from build123d import *

# Parameters (mm, degrees)
SKETCH_1_R           = 3.5
EXTRUDE_1_DEPTH      = 3
SKETCH_2_R           = 1.5
CUT_EXTRUDE_1_DEPTH  = 10
EXTRUDE_2_DEPTH      = 4
EXTRUDE_5_DEPTH      = 7
FILLET_1_R           = 2
HOLE_WIZARD_M2_5_1_D = 2.05
SKETCH_12_R          = 4.953561737
SKETCH_12_R_2        = 3.03
EXTRUDE_6_DEPTH      = 3


with BuildPart() as part:
    # 草图1 → 凸台-拉伸1 (new body)
    with BuildSketch(Plane.XY):
        with BuildLine():
            Line((0, 0), (17, 0))
            Line((17, 0), (17, 21))
            ThreePointArc((17, 21), (14.559389791, 26.961023013), (8.639106973, 29.498861644))
            ThreePointArc((8.639106973, 29.498861644), (4.214678609, 30.921411086), (1.327625741, 34.563407653))
            ThreePointArc((1.327625741, 34.563407653), (-5.234705957, 62.223549547), (-3.748501306, 90.612611571))
            ThreePointArc((-3.748501306, 90.612611571), (-5.162788524, 92.923505905), (-7.58241645, 91.704554856))
            ThreePointArc((-7.58241645, 91.704554856), (-12.196269834, 55.45091149), (0, 21))
            Line((0, 21), (0, 0))
        make_face()
        with Locations((8.5, 21)):
            Circle(SKETCH_1_R, mode=Mode.SUBTRACT)
    extrude(amount=EXTRUDE_1_DEPTH)

    # 草图2 → 切除-拉伸1 (cut)
    with BuildSketch(Plane(origin=(0, 0, 0), x_dir=(-1, 0, 0), z_dir=(0, 0, -1))):
        with Locations((-14, 4)):
            Circle(SKETCH_2_R)
        with Locations(Location((-3, 4, 0), (0, 0, 180))):
            Circle(SKETCH_2_R)
    extrude(amount=-CUT_EXTRUDE_1_DEPTH, mode=Mode.SUBTRACT)

    # 草图3 → 凸台-拉伸2 (add)
    with BuildSketch(Plane.XY.offset(3)):
        with BuildLine():
            ThreePointArc((-7.58241645, 91.704554856), (-12.6426678, 63.080202535), (-7.007767698, 34.563407653))
            Line((-7.007767698, 34.563407653), (1.327625741, 34.563407653))
            ThreePointArc((1.327625741, 34.563407653), (-5.234705957, 62.223549547), (-3.748501306, 90.612611571))
            ThreePointArc((-3.748501306, 90.612611571), (-5.162788524, 92.923505905), (-7.58241645, 91.704554856))
        make_face()
    extrude(amount=EXTRUDE_2_DEPTH)

    # 草图8 → 凸台-拉伸5 (add)
    with BuildSketch(Plane(origin=(0, 0, 0), x_dir=(-1, 0, 0), z_dir=(0, 0, -1))):
        with BuildLine():
            Line((8.353336216, 89.563407653), (13.622203114, 89.563407653))
            ThreePointArc((13.622203114, 89.563407653), (17.624786926, 61.957713987), (12.366747323, 34.563407653))
            Line((12.366747323, 34.563407653), (7.007767698, 34.563407653))
            ThreePointArc((7.007767698, 34.563407653), (12.623031035, 61.942490485), (8.353336216, 89.563407653))
        make_face()
    extrude(amount=-EXTRUDE_5_DEPTH)

    # 圆角1
    fillet_1_edges = [part.edges().sort_by_distance(p)[0] for p in [
        (-12.366747323, 34.563407653, 3.5),
        (-13.622203114, 89.563407653, 3.5),
        (-8.353336216, 89.563407653, 3.5),
        (-7.007767698, 34.563407653, 1.5),
    ]]
    fillet(fillet_1_edges, radius=FILLET_1_R)

    # M2.5 螺纹孔1 (through all)
    with Locations(Plane(origin=(0, 0, 0), x_dir=(-1, 0, 0), z_dir=(0, 0, -1))):
        with Locations((14.33753876, 52.418963936), (-20.3596947, 65.689324708), (13.008857265, 82.418963936), (15.069556912, 67.418963936)):
            Hole(HOLE_WIZARD_M2_5_1_D / 2)

    # 草图12 → 凸台-拉伸6 (add)
    with BuildSketch(Plane(origin=(0, 0, 0), x_dir=(-1, 0, 0), z_dir=(0, 0, -1))):
        with Locations((-8.5, 21)):
            Circle(SKETCH_12_R)
        with Locations((-8.5, 21)):
            Circle(SKETCH_12_R_2, mode=Mode.SUBTRACT)
    extrude(amount=-EXTRUDE_6_DEPTH)


solid = part.part
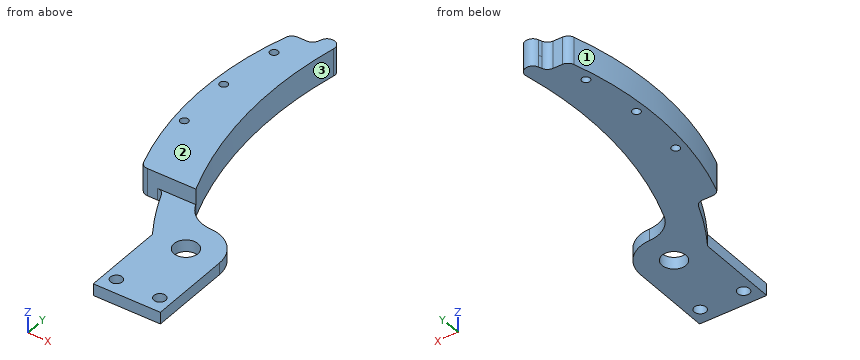
Design review of the part built by this model. Coordinates are the model's own, in mm. Face numbers are marked on the shaded views. Round coordinates to 2 decimals unless told otherwise and drop trailing zeros. Order: outer loops, then holes, each group sorted by start corner. A loop starts at its lowest first (then second) coordinate and runs counter-clockwise, first axis right, second up.
1) Consider section A-A (y = 4). State the section outline as (x, z) points.
The answers:
outline: (0, 0) - (1.5, 0) - (1.5, 3) - (0, 3) - close; (4.5, 0) - (12.5, 0) - (12.5, 3) - (4.5, 3) - close; (15.5, 0) - (17, 0) - (17, 3) - (15.5, 3) - close
2) Consider section B-B (x = 14). State the section outline as (y, z) points, plus the area to 3 significant figures.
The answers:
outline: (0, 0) - (2.5, 0) - (2.5, 3) - (0, 3) - close; (5.5, 0) - (27.48, 0) - (27.48, 3) - (5.5, 3) - close
area: 73.4 mm2
3) For L1, parallel to Y at x = -8, z = 3.5; L2, parallel to Y at x = 8.5, z = 2; L3, parallel to Y at x = 3, z = 1.15, list the stretches that pass through material, from the lowest coordinate up.
The answers:
L1: y = 34.56 to 90.63
L2: y = 0 to 17.97, 24.03 to 29.5
L3: y = 0 to 2.5, 5.5 to 31.96
4) Consider section D-D (x = 2.5). State the section outline as (y, z) points.
The answers:
outline: (0, 0) - (2.59, 0) - (2.59, 3) - (0, 3) - close; (5.41, 0) - (32.53, 0) - (32.53, 3) - (5.41, 3) - close
5) Draft analysis for pull direction Y (two halves, no side actions). For the marked faces 1, 2 and 3, state which applies: released by +Y, released by -Y, zero draft, split by the parting line, or undercut.
The answers:
face 1: split by the parting line
face 2: zero draft
face 3: undercut
6) Consider section C-C (z = 4.25). Count the separate pieces of the cut face and the enclosed holes in it, plus the area to 3 significant figures.
The answers:
separate pieces: 1
enclosed holes: 3
area: 672 mm2
7) Clearance check with flat-ended pins moving along their axes: pin 1 Ø0.7 at (x, z) = (-10.5, 2) entering from +Y; pin 2 Ø4 at (x, z) = (-1, 5.5) entering from -Y; pin 3 Ø1.5 at (y, z) = (8, 2) entering from -X; pin 4 Ø2.5 at (x, y) = (-13.01, 82.42) entering from +Z. State where each tip first meets the part, or that it passes through.
The answers:
pin 1: stops at y = 89.56
pin 2: stops at y = 34.56
pin 3: stops at x = 0
pin 4: stops at z = 7
